Verification items for the finished model (mm, model axes). Give positions to 0.01 mm unless a question says otherwise; leave off trailing zeros. Order: outer loops, then holes, each group sorted by start corner. A loop starts at its lowest first (then second) coordinate and runs counter-clockwise, first axis right, second up. Notation, with made-up numbers: (42, 77) -> (54, 77) arc R23 cw to (54, 93) -> close; hole circle Ø3 at (34, -4). An arc over 180 degrees is marked (long way). Return JSON: item names as keys, results as strings. Group by question number.
(1) Thickness scan on line 1 along Y through (x, z) = (1.75, 1.3); line 2 along X through (y, z) = (-2, -0.2); line 3 along Z through (x, y) = (1.7, -19.5). Record the ranges inside material, lowest first.
(2) Depth check by flat-ended pin: pin 1 Ø1.3 at (x, z) = (-0.5, -1) entering from -Y; pin 2 Ø2 at (x, y) = (-1.5, -2) entering from +Z; pin 3 Ø2 at (x, y) = (-1, -18.5) entering from -Z. Enter the tip coordinate at first touch or a pass-through.
(3) Cross-section at C-C on z = 1.75. Enter the section's corners in (x, y).
(4) Cross-section at A-A on y = -1.5. Enter the section's corners in (x, z), then the cut area to 3 significant figures.
(5) Cross-section at B-B on x = 0.75. Enter the section's corners in (y, z), then the cut area to 3 significant figures.
from build123d import *

# Parameters (mm, degrees)
BOSS_EXTRUDE1_DEPTH = 2.4
SKETCH2_R           = 0.25
BOSS_EXTRUDE2_DEPTH = 34


with BuildPart() as part:
    # Sketch1 → Boss-Extrude1 (new body)
    with BuildSketch(Plane(origin=(0, 0, 0), x_dir=(1, 0, 0), z_dir=(0, 1, 0))):
        with BuildLine():
            ThreePointArc((2.55, 0), (2.235943184, 1.22599269), (1.37113092, 2.15))
            Line((1.37113092, 2.15), (-1.37113092, 2.15))
            ThreePointArc((-1.37113092, 2.15), (-2.235943184, 1.22599269), (-2.55, 0))
            ThreePointArc((-2.55, 0), (-2.235943184, -1.22599269), (-1.37113092, -2.15))
            Line((-1.37113092, -2.15), (1.37113092, -2.15))
            ThreePointArc((1.37113092, -2.15), (2.235943184, -1.22599269), (2.55, 0))
        make_face()
    extrude(amount=BOSS_EXTRUDE1_DEPTH)

    # Sketch2 → Boss-Extrude2 (add)
    with BuildSketch(Plane.XZ):
        with Locations(Location((-1.7, 0, 0), (0, 0, 90))):
            Circle(SKETCH2_R)
        with Locations(Location((1.7, 0, 0), (0, 0, 90))):
            Circle(SKETCH2_R)
    extrude(amount=BOSS_EXTRUDE2_DEPTH)


solid = part.part
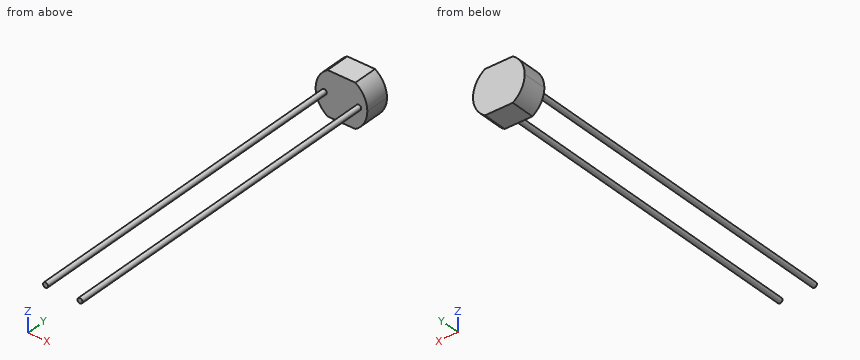
Verdict:
{
 "1": {"line 1": "0 to 2.4", "line 2": "-1.85 to -1.55, 1.55 to 1.85", "line 3": "-0.25 to 0.25"},
 "2": {"pin 1": "y = 0", "pin 2": "z = 0.25", "pin 3": "z = -0.25"},
 "3": {"outline": "(-1.85, 0) -> (1.85, 0) -> (1.85, 2.4) -> (-1.85, 2.4) -> close"},
 "4": {"outline": "circle Ø0.5 at (-1.7, 0); circle Ø0.5 at (1.7, 0)", "area": "0.393 mm²"},
 "5": {"outline": "(0, -2.15) -> (2.4, -2.15) -> (2.4, 2.15) -> (0, 2.15) -> close", "area": "10.3 mm²"}
}
